The listing builds one solid part. Answer for the finished solid, in the listing's coordinates (mm). A direction names the side the tool comes from. Give positions to 0.01 mm unless a question says otherwise; leave off trailing zeros. Write each loop counter-clockwise with the first axis right and the second up, starting at its lowest first coordinate (ties: lowest second). Pieces come first, ordered by that corner, then holes. Notation, with made-up numbers: M 58.5,85.5 L 73.5,85.5 A30 ccw 73.5,123.5 Z; hole C 45,72.25 d6. An arc over 180 degrees is marked long. Return JSON: item names as keys, results as strings.
from build123d import *

# Parameters (mm, degrees)
F1_DEPTH = 80
F2_W     = 189.999994
F2_H     = 143.999994
F3_DEPTH = 75
F4_R     = 16
F5_DEPTH = 200.001


with BuildPart() as f1:
    # F0 (on Top) → F1 (new body)
    with BuildSketch(Plane.XY):
        with BuildLine():
            ThreePointArc((100, 72), (98.535534, 75.535534), (95, 77))
            Line((95, 77), (-95, 77))
            ThreePointArc((-95, 77), (-98.535534, 75.535534), (-100, 72))
            Line((-100, 72), (-100, -72))
            ThreePointArc((-100, -72), (-98.535534, -75.535534), (-95, -77))
            Line((-95, -77), (95, -77))
            ThreePointArc((95, -77), (98.535534, -75.535534), (100, -72))
            Line((100, -72), (100, 72))
        make_face()
    extrude(amount=F1_DEPTH)

    # F2 (on face) → F3 (cut)
    with BuildSketch(Plane.XY.offset(80)):
        Rectangle(F2_W, F2_H)
    extrude(amount=-F3_DEPTH, mode=Mode.SUBTRACT)

    # F4 (on face) → F5 (cut, through all)
    with BuildSketch(Plane.YZ.offset(100)):
        with Locations((26, 27)):
            Circle(F4_R)
        with Locations((-26, 27)):
            Circle(F4_R)
    extrude(amount=-F5_DEPTH, mode=Mode.SUBTRACT)


solid = f1.part
Item 1: A cutting plane is placed at B-B, the plane z = 27. Write down the section's boundary in (x, y), plus the area to 3 significant figures.
Geometry results:
{"outline": "M -100,-72 A5 ccw -95,-77 L 95,-77 A5 ccw 100,-72 L 100,-42 L 95,-42 L 95,-72 L -95,-72 L -95,-42 L -100,-42 Z; M -100,-10 L -95,-10 L -95,10 L -100,10 Z; M -100,42 L -95,42 L -95,72 L 95,72 L 95,42 L 100,42 L 100,72 A5 ccw 95,77 L -95,77 A5 ccw -100,72 Z; M 95,-10 L 100,-10 L 100,10 L 95,10 Z", "area": "2,780 mm2"}
Item 2: Determine the mould class of faces 1 (the flat face through (-95, -1, 43)), 2 (the cylindrical face through (97.53, -10.74, 31.81)), 3 (the cylindrical face through (98, -76, 39)) for opening direction X: +X half, -X half, draft (parallel to the pull), parting line (faces both ways), or undercut.
Geometry results:
{"face 1": "undercut", "face 2": "draft", "face 3": "+X half"}
Item 3: A cutting plane is placed at A-A, the plane y = 26. Write down the section's boundary in (x, z).
Geometry results:
{"outline": "M -100,0 L 100,0 L 100,11 L 95,11 L 95,5 L -95,5 L -95,11 L -100,11 Z; M -100,43 L -95,43 L -95,80 L -100,80 Z; M 95,43 L 100,43 L 100,80 L 95,80 Z"}
Item 4: Find the intervals of material crossed by line 1 (Y direction, x = 80.5, z = 61.5); line 2 (X direction, y = -50, z = 67); line 3 (Z direction, x = -96, y = 26), in increasing order.
Geometry results:
{"line 1": "y = -77 to -72, 72 to 77", "line 2": "x = -100 to -95, 95 to 100", "line 3": "z = 0 to 11, 43 to 80"}
Item 5: Which of the six approach directions +Z, -Z, +X, -X, +Y, -Y give full straight-line access (tool end or side, diameter ignored) to faces 4 (the cylindrical face through (97.53, 41.26, 31.81)), 5 (the flat face through (-1, 72, 43))?
Geometry results:
{"face 4": "+X, -X", "face 5": "+Z"}
Item 6: A cutting plane is placed at C-C, the plane y = 58. Write down the section's boundary in (x, z), plus the area to 3 significant figures.
Geometry results:
{"outline": "M -100,0 L 100,0 L 100,80 L 95,80 L 95,5 L -95,5 L -95,80 L -100,80 Z", "area": "1,750 mm2"}
Item 7: A cutting plane is placed at D-D, the plane z = 69.5. Write down the section's boundary in (x, y), plus the area to 3 significant figures.
Geometry results:
{"outline": "M -100,-72 A5 ccw -95,-77 L 95,-77 A5 ccw 100,-72 L 100,72 A5 ccw 95,77 L -95,77 A5 ccw -100,72 Z; hole M -95,-72 L 95,-72 L 95,72 L -95,72 Z", "area": "3,420 mm2"}
Item 8: Given pin 1 Ø12 at (x, y) = (71.5, -3.5) entering from +Z; pin 2 Ø19 at (y, z) = (-26, 27) entering from +X, each flat-ended and moving along its own axis, determine where each tip first touches the part or whether it passes through.
Geometry results:
{"pin 1": "stops at z = 5", "pin 2": "passes through"}
